Design review of the part built by this model. Coordinates are the model's own, in mm. A direction names the side the tool comes from. Coordinates: 2 decimals unless noted, no trailing zeros. Loops run counter-clockwise (first coordinate to the right, second up) from the corner with the lowest first, then second, coordinate; pieces in that order, holes last. Notation, with made-up numbers: M -26,70 L -22,70 A14 ccw -22,76 Z; hole C 27.25,35.5 d4. An arc over 180 degrees is marked long. Answer as a JSON object with one key per item and string values. Group by question number.
1. To check wall thickness, follow probe 1 along Z at (x, y) = (107.5, 50.5); probe 2 along Y at (x, z) = (128, 3); probe 3 along Y at (x, z) = (39, -46.5). State the ranges of each line that lie inside material, in increasing order.
2. Consider section A-A (y = 35.5). State the section outline as (x, z) points.
3. Draft analysis for pull direction Z (two halves, no side actions). For faces 6 (the flat face through (87, 16, 65.8)), 7 (the flat face through (88, 60, -75)), 8 (the flat face through (88, 28, -81.2)), 9 (the flat face through (88, 28, 102.8)), state which applies: +Z half, -Z half, draft (parallel to the pull), parting line (faces both ways), or undercut.
4. Consider section B-B (x = 90). State the section outline as (y, z) points.
5. Consider section C-C (x = 19). State the section outline as (y, z) points.
6. Insertion check: pin 1 (6 mm diameter, centred on y = 17.5, z = -50, fed in from -X); pin 2 (7.5 mm diameter, centred on x = 89.5, z = -55, fed in from +Y); pin 3 (5 mm diameter, centred on x = 159, z = 11.5, fed in from +Y). Each pin has a flat end and moves straight along its axis. Give the tip position at first contact, or say it passes through.
7. Machinability: for faces 1 (the flat face through (88, 41, -69.2)), 2 (the flat face through (85, -5, 12)), 3 (the cylindrical face through (86.92, 23.85, -66.19)), 4 (the flat face through (36.16, 17, 76)), 5 (the flat face through (136.16, 17, -55)), which of the approach directions +Z, -Z, +X, -X, +Y, -Y give a long, thin tool a straight path to every point of the face, cutting with its end or side? Answer none if there is none.
8. Consider section D-D (z = -36). State the section outline as (x, y) points.
Autodesk Inventor part; units mm, degrees
ref_plane "YZ Plane" through (0, 0, 0) normal (1, 0, 0) x (0, 1, 0)
ref_plane "XZ Plane" through (0, 0, 0) normal (0, 1, 0) x (-1, 0, 0)
ref_plane "XY Plane" through (0, 0, 0) normal (0, 0, 1) x (1, 0, 0)
sketch "Sketch1" plane through (0, 0, 0) normal (0, 1, 0) x (-1, 0, 0)
  line L0 (13.84, 90.8) -> (-186.16, 90.8)
  line L1 (-186.16, 90.8) -> (-186.16, -69.2)
  line L2 (-186.16, -69.2) -> (13.84, -69.2)
  line L3 (13.84, -69.2) -> (13.84, 90.8)
  point P0 (0, 0)
  dimension "d0" = 160
  dimension "d1" = 200
extrude "Extrusion1" add sketch "Sketch1" along normal blind 11
sketch "Sketch2" plane through (186.16, 0, 90.8) normal (1, 0, 0) x (0, 0, -1)
  line L0 (0, 0) -> (0, 11)
  line L1 (0, 0) -> (-12, 0)
  line L2 (-12, 0) -> (-12, 60)
  line L3 (-12, 60) -> (0, 60)
  line L4 (0, 60) -> (0, 0)
  line L5 (160, 0) -> (160, 11)
  line L6 (160, 0) -> (172, 0)
  line L7 (172, 0) -> (172, 60)
  line L8 (172, 60) -> (160, 60)
  line L9 (160, 60) -> (160, 0)
  point P0 (90.8, 0)
  point P1 (0, 11)
  dimension "d4" = 60
  dimension "d5" = 60
  dimension "d6" = 12
  dimension "d17" = 12
extrude "Extrusion2" add sketch "Sketch2" against normal up to surface (200 mm away)
sketch "Sketch3" plane through (0, 0, 0) normal (0, -1, 0) x (1, 0, 0)
  line L0 (186.16, 102.8) -> (186.16, -81.2)
  line L1 (186.16, 102.8) -> (-13.84, 102.8)
  line L2 (-13.84, -81.2) -> (-13.84, 102.8)
  line L3 (186.16, -81.2) -> (-13.84, -81.2)
  point P0 (0, 0)
extrude "Extrusion3" add sketch "Sketch3" along normal blind 5
sketch "Sketch7" plane through (0, 11, 0) normal (0, 1, 0) x (1, 0, 0)
  line L0 (186.16, -90.8) -> (-13.84, -90.8)
  line L1 (36.16, -90.8) -> (136.16, -90.8)
  line L2 (136.16, -90.8) -> (136.16, -65.8)
  line L3 (136.16, -65.8) -> (36.16, -65.8)
  line L4 (36.16, -65.8) -> (36.16, -90.8)
  line L5 (186.16, 69.2) -> (-13.84, 69.2)
  line L6 (36.16, 69.2) -> (136.16, 69.2)
  line L7 (136.16, 69.2) -> (136.16, 44.2)
  line L8 (136.16, 44.2) -> (36.16, 44.2)
  line L9 (36.16, 44.2) -> (36.16, 69.2)
  line L10 (-13.84, 69.2) -> (-13.84, -90.8)
  line L11 (186.16, -90.8) -> (186.16, 69.2)
  point P0 (0, 0)
  point P1 (136.16, 56.7)
  dimension "d18" = 25
  dimension "d19" = 25
  dimension "d20" = 50
  dimension "d21" = 50
  dimension "d22" = 50
  dimension "d23" = 50
extrude "Extrusion6" add sketch "Sketch7" along normal blind 10 contours L0 L4 L3 L2 | L7 L8 L9 L5
fillet "Fillet1" radius 4 4 edges at (36.16, 16, -69.2) (36.16, 16, 90.8) (136.16, 16, -69.2) (136.16, 16, 90.8)
fillet "Fillet2" radius 10 4 edges at (138.16, 21, -69.2) (34.16, 21, -69.2) (34.16, 21, 90.8) (138.16, 21, 90.8)
sketch "Sketch8" plane through (-13.84, 11, 90.8) normal (-1, 0, 0) x (0, 0, 1)
  line L0 (-160, 0) -> (0, 0)
  line L1 (0, 0) -> (0, -19)
  line L2 (0, -19) -> (-160, -19)
  line L3 (-160, -19) -> (-160, 0)
  line L4 (-172, 49) -> (12, 49)
  line L5 (12, 49) -> (12, -16)
  line L6 (12, -16) -> (-172, -16)
  line L7 (-172, -16) -> (-172, 49)
  point P0 (-90.8, -11)
properties part number "Y_karetka" material "Aluminum 6061"
Findings below:
{
 "1": {"probe 1": "z = -81.2 to -69.2, 90.8 to 102.8", "probe 2": "y = -5 to 11", "probe 3": "y = -5 to 21"},
 "2": {"outline": "M -13.84,-81.2 L 186.16,-81.2 L 186.16,-69.2 L -13.84,-69.2 Z; M -13.84,90.8 L 186.16,90.8 L 186.16,102.8 L -13.84,102.8 Z"},
 "3": {"face 6": "undercut", "face 7": "draft", "face 8": "-Z half", "face 9": "+Z half"},
 "4": {"outline": "M -5,-81.2 L 60,-81.2 L 60,-69.2 L 31,-69.2 A10 cw 21,-59.2 L 21,-44.2 L 11,-44.2 L 11,65.8 L 21,65.8 L 21,80.8 A10 cw 31,90.8 L 60,90.8 L 60,102.8 L -5,102.8 Z"},
 "5": {"outline": "M -5,-81.2 L 60,-81.2 L 60,-69.2 L 11,-69.2 L 11,90.8 L 60,90.8 L 60,102.8 L -5,102.8 Z"},
 "6": {"pin 1": "stops at x = 36.16", "pin 2": "stops at y = 21", "pin 3": "stops at y = 11"},
 "7": {"face 1": "+Y", "face 2": "+Z, -Z, +X, -X, -Y", "face 3": "+X, -X, +Y", "face 4": "-X, +Y", "face 5": "+X, +Y"},
 "8": {"outline": "M -13.84,-5 L 186.16,-5 L 186.16,11 L -13.84,11 Z"}
}
